from build123d import *

# Parameters (mm, degrees)
BOSS_EXTRUDE1_DEPTH = 2.032
FILLET1_R           = 3
FILLET2_R           = 2
SKETCH14_R          = 1.5874999999999986
CUT_EXTRUDE1_DEPTH  = 70.16809880796494
SKETCH15_W          = 14.760000000000002
SKETCH15_H          = 12.699999999999996
BOSS_EXTRUDE4_DEPTH = 2.032
EDGE_FLANGE3_DEPTH  = 14.760000000000002
BOSS_EXTRUDE5_DEPTH = 2.032
EDGE_FLANGE4_DEPTH  = 14.760000000000002
FILLET4_R           = 2.38125


# Sheet-metal steps are written as plain solids
with BuildPart() as part:
    # Sketch3 → Boss-Extrude1 (new body)
    with BuildSketch(Plane.XY):
        with BuildLine():
            ThreePointArc((4.574999999999999, 10.775), (9.225864227432316, 16.77834726283189), (16.200863986500366, 13.774999999999732))
            Line((16.20086398650046, 13.774999999999999), (28.34913601349985, 13.774999999999999))
            ThreePointArc((28.349136013499827, 13.775000000000073), (33.77500000000019, 16.974999999999998), (39.20086398650036, 13.77499999999973))
            Line((39.20086398650045, 13.774999999999999), (51.34913601349986, 13.774999999999999))
            ThreePointArc((51.34913601349983, 13.775000000000077), (58.32413577256787, 16.778347262831836), (62.974999999999994, 10.775000000000002))
            Line((62.974999999999994, 10.775), (62.975, 28.534999999999997))
            Line((62.97500000000001, 28.534999999999997), (4.574999999999999, 28.534999999999997))
            Line((4.574999999999999, 28.534999999999997), (4.574999999999999, 10.774999999999999))
        make_face()
    extrude(amount=BOSS_EXTRUDE1_DEPTH)

    # Fillet1
    fillet1_edges = [part.edges().sort_by_distance(p)[0] for p in [
        (4.574999999999999, 28.534999999999997, 1.016),
        (62.97500000000001, 28.534999999999997, 1.016),
    ]]
    fillet(fillet1_edges, radius=FILLET1_R)

    # Fillet2
    fillet2_edges = [part.edges().sort_by_distance(p)[0] for p in [
        (62.974999999999994, 10.775000000000002, 1.016),
    ]]
    fillet(fillet2_edges, radius=FILLET2_R)
    fillet2_2_edges = [part.edges().sort_by_distance(p)[0] for p in [
        (51.349136013499844, 13.775000000000038, 1.016),
    ]]
    fillet(fillet2_2_edges, radius=FILLET2_R)
    fillet2_3_edges = [part.edges().sort_by_distance(p)[0] for p in [
        (39.20086398650041, 13.774999999999864, 1.016),
    ]]
    fillet(fillet2_3_edges, radius=FILLET2_R)
    fillet2_4_edges = [part.edges().sort_by_distance(p)[0] for p in [
        (28.349136013499837, 13.775000000000036, 1.016),
    ]]
    fillet(fillet2_4_edges, radius=FILLET2_R)
    fillet2_5_edges = [part.edges().sort_by_distance(p)[0] for p in [
        (4.574999999999999, 10.774999999999999, 1.016),
    ]]
    fillet(fillet2_5_edges, radius=FILLET2_R)
    fillet2_6_edges = [part.edges().sort_by_distance(p)[0] for p in [
        (16.200863986500412, 13.774999999999865, 1.016),
    ]]
    fillet(fillet2_6_edges, radius=FILLET2_R)

    # Sketch14 → Cut-Extrude1 (cut, through all)
    with BuildSketch(Plane(origin=(0, 0, 0), x_dir=(-1, 0, 0), z_dir=(0, 0, -1))):
        with Locations((-45.275, 22.184999999999995)):
            Circle(SKETCH14_R)
        with Locations((-22.275000000000002, 22.184999999999995)):
            Circle(SKETCH14_R)
    extrude(amount=-CUT_EXTRUDE1_DEPTH, mode=Mode.SUBTRACT)

    # Sketch15 → Boss-Extrude4 (add)
    with BuildSketch(Plane.XY.offset(2.032)):
        with Locations((36.545, 34.88499999999999)):
            Rectangle(SKETCH15_W, SKETCH15_H)
    extrude(amount=-BOSS_EXTRUDE4_DEPTH)

    # Edge-Flange3 section (across the edge) → Edge-Flange3 (add)
    with BuildSketch(Plane(origin=(29.165000000000003, 43.266999999999996, 1.419e-14), x_dir=(0, -1, -3.49e-15), z_dir=(1, 0, 0))):
        with BuildLine():
            Line((-2.032, 2.032000000000007), (-2.032, 42.418000000000006))
            Line((-2.032, 42.418000000000006), (0, 42.418000000000006))
            Line((0, 42.418000000000006), (0, 2.032000000000007))
            ThreePointArc((0, 2.032000000000007), (0.5951590206289381, 0.5951590206289399), (2.032000000000007, 7.11e-15))
            Line((2.032000000000007, 7.11e-15), (2.0320000000000142, -2.031999999999993))
            ThreePointArc((2.0320000000000142, -2.031999999999993), (-0.8416819587421238, -0.8416819587421274), (-2.032, 2.032000000000007))
        make_face()
    extrude(amount=EDGE_FLANGE3_DEPTH)

    # Sketch19 → Boss-Extrude5 (add)
    with BuildSketch(Plane(origin=(0, 45.298999999999985, 1.5561e-13), x_dir=(1, 0, 0), z_dir=(0, 1, 3.44e-15))):
        Polygon((29.165000000000003, 42.41800000000015), (17.735000000000003, 42.41800000000015), (17.73500000000001, 27.658000000000147), (29.165000000000006, 27.658000000000147), align=None)
    extrude(amount=-BOSS_EXTRUDE5_DEPTH)

    # Edge-Flange4 section (across the edge) → Edge-Flange4 (add)
    with BuildSketch(Plane(origin=(15.703000000000005, 43.2670000000001, -27.657999999999998), x_dir=(1, -3.49e-15, -4.7e-16), z_dir=(-4.7e-16, 3.29e-15, -1))):
        with BuildLine():
            Line((-2.032, 2.032000000000007), (-2.032, 11.93800000000001))
            Line((-2.032, 11.93800000000001), (0, 11.93800000000001))
            Line((0, 11.93800000000001), (0, 2.032000000000007))
            ThreePointArc((0, 2.032000000000007), (0.5951590206289381, 0.5951590206289399), (2.032000000000007, 7.11e-15))
            Line((2.032000000000007, 7.11e-15), (2.0320000000000142, -2.031999999999993))
            ThreePointArc((2.0320000000000142, -2.031999999999993), (-0.8416819587421238, -0.8416819587421274), (-2.032, 2.032000000000007))
        make_face()
    extrude(amount=EDGE_FLANGE4_DEPTH)

    # Fillet4
    fillet4_edges = [part.edges().sort_by_distance(p)[0] for p in [
        (29.165000000000006, 44.28300000000008, -27.657999999999994),
        (29.165000000000003, 28.534999999999997, 1.016),
        (43.925000000000004, 28.534999999999997, 1.016),
        (43.925000000000004, 44.28300000000014, -42.41799999999999),
    ]]
    fillet(fillet4_edges, radius=FILLET4_R)


solid = part.part
CAD build for the part. Positions are in the model's coordinates, mm. A direction names the side the tool comes from. Coordinates: 2 decimals unless noted, no trailing zeros. Order: outer loops, then holes, each group sorted by start corner. A loop starts at its lowest first (then second) coordinate and runs counter-clockwise, first axis right, second up. Notation, with made-up numbers: (-11.5, 82.5) -> (34.5, 82.5) arc R24 cw to (34.5, 118.5) -> close; hole circle Ø5 at (-23, -10.5). An arc over 180 degrees is marked (long way). Answer in a Markdown table with one row per item.
1) Band-saw the part on A-A (y = 39). List the corners of the cut face in (x, z) (3 decimals).
Check values:
| item | result |
|---|---|
| outline | (13.671, -42.418) -> (15.703, -42.418) -> (15.703, -27.658) -> (13.671, -27.658) -> close; (29.165, 0) -> (43.925, 0) -> (43.925, 2.032) -> (29.165, 2.032) -> close |
2) Band-saw the part on D-D (y = 23). List the corners of the cut face in (x, z) (3 decimals).
Check values:
| item | result |
|---|---|
| outline | (4.575, 0) -> (20.913, 0) -> (20.913, 2.032) -> (4.575, 2.032) -> close; (23.637, 0) -> (43.913, 0) -> (43.913, 2.032) -> (23.637, 2.032) -> close; (46.637, 0) -> (62.975, 0) -> (62.975, 2.032) -> (46.637, 2.032) -> close |
3) Band-saw the part on C-C (z = -32). List the corners of the cut face in (x, y) (3 decimals).
Check values:
| item | result |
|---|---|
| outline | (13.671, 31.329) -> (15.703, 31.329) -> (15.703, 41.235) arc R2.032 cw to (17.735, 43.267) -> (43.925, 43.267) -> (43.925, 45.299) -> (17.735, 45.299) arc R4.064 ccw to (13.671, 41.235) -> close |
4) Mould opens along X. For faces 4 (the face through (14.893, 44.14, -34.935)), 5 (the face through (62, 16.1, 1)), 6 (the face through (34, 43.267, -27)) say: pulls with the +X half, pulls with the -X half, needs draft (parallel to the pull), parting line crosses it, or undercut.
Check values:
| item | result |
|---|---|
| face 4 | pulls with the -X half |
| face 5 | undercut |
| face 6 | needs draft |
5) Flat gauge pins, fed straight in: P1, Ø13, axis at x = 30.5, z = -15, coming from the -Y side; P2, Ø4.5, axis at y = 40.5, z = -29, coming from the +X side; P3, Ø11.5, axis at y = 35.5, z = -18, coming from the -X side; P4, Ø3, axis at y = 36.5, z = -32.5, coming from the -X side. Where does each tip first touch, or does it go through?
Check values:
| item | result |
|---|---|
| P1 | y = 43.27 |
| P2 | x = 16.38 |
| P3 | through |
| P4 | x = 13.67 |
6) Which spindle directions (+Z, -Z, +X, -X, +Y, -Y) get a long thin tool onto all of the face, cutting with end or side? Do faces 1 (the face through (16.282, 42.656, -34.935)), 2 (the face through (39.402, 13.975, 1.03)), 3 (the face through (17, 28.535, 1)). Say none if no direction does.
Check values:
| item | result |
|---|---|
| face 1 | +Z, -Z, +X, -Y |
| face 2 | +Z, -Z, -Y |
| face 3 | +Z, -Z, -X, +Y |
7) Band-saw the part on B-B (x = 45). List the corners of the cut face in (y, z) (1 decimal).
Check values:
| item | result |
|---|---|
| outline | (13.8, 0) -> (20.6, 0) -> (20.6, 2) -> (13.8, 2) -> close; (23.7, 0) -> (28.9, 0) -> (28.9, 2) -> (23.7, 2) -> close |
8) Drill centre lines: line 1 (Z direction, x = 26, y = 28); line 2 (Y direction, x = 42, z = -8.5); line 3 (X direction, y = 33, z = -36). Where is each one in solid material? Low to high.
Check values:
| item | result |
|---|---|
| line 1 | 0 to 2.03 |
| line 2 | 43.27 to 45.3 |
| line 3 | 13.67 to 15.7 |
